Here's the drawing with two shaded views (mm, measured from the low corner). I have some questions. Coordinates: 2 decimals unless noted, no trailing zeros. Write each loop counter-clockwise with the first axis right and the second up, starting at its lowest first coordinate (ties: lowest second). Pieces come first, ordered by that corner, then holes.
Item 1: I want a section at A-A on y = 80.5. Please give me the cut outline in (x, z) (1 decimal).
Item 2: For P1, Ø0.9, axis at y = 75.5, z = 2, coming from the -X side (1 decimal); P2, Ø7, axis at x = 4, y = 23.35, coming from the +Z side; P3, Ø0.9, axis at y = 84, z = 1.5, coming from the +X side, each with a flat end and sliding along its axis, tell me the tip position at first contact or that it passes through.
Item 3: I want a section at B-B on x = 139. Please give me the cut outline in (y, z).
Item 4: If I drill on probe 1 along Y at (x, z) = (155, 1.6) (1 decimal); probe 2 along X at (y, z) = (36.5, 0.25) (1 decimal); probe 3 along X at (y, z) = (42, 1.9) (1 decimal), over which ranges is the centre line in solid material (lowest first)?
Item 5: I want a section at C-C on z = 1.6. State how many separate pieces and enclosed holes the cut face has, then the cut area to 3 significant figures.
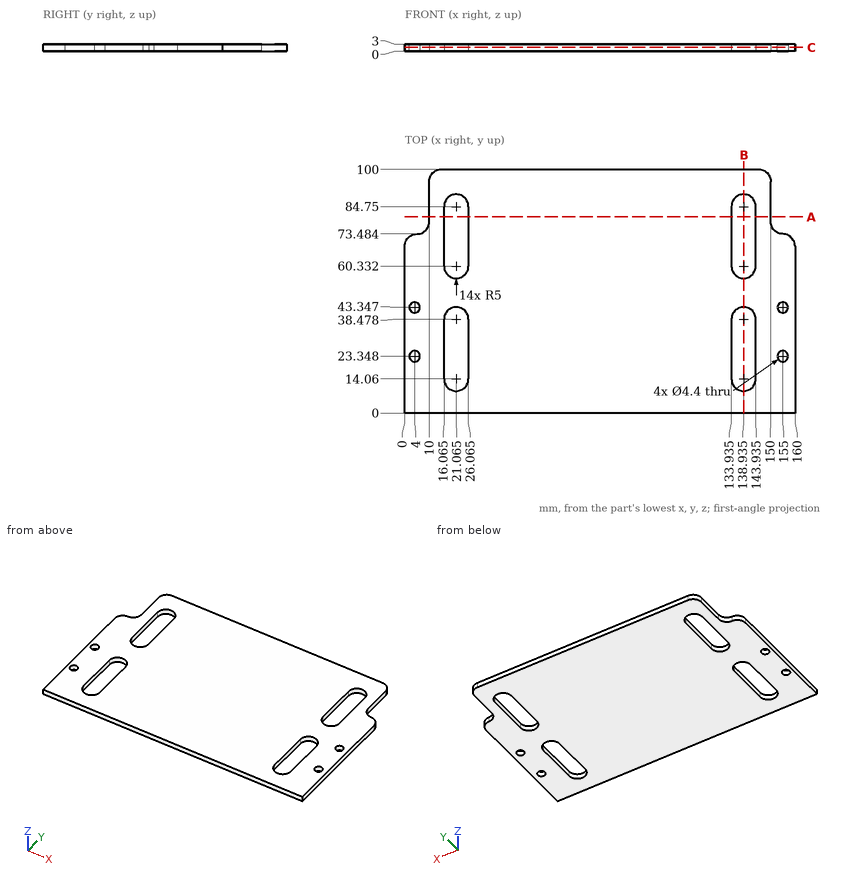
Response values:
1. outline: (10, 0) - (16.1, 0) - (16.1, 3) - (10, 3) - close; (26.1, 0) - (133.9, 0) - (133.9, 3) - (26.1, 3) - close; (143.9, 0) - (150, 0) - (150, 3) - (143.9, 3) - close
2. P1: stops at x = 8.6
2. P2: stops at z = 3
2. P3: stops at x = 150
3. outline: (0, 0) - (9.06, 0) - (9.06, 3) - (0, 3) - close; (43.48, 0) - (55.33, 0) - (55.33, 3) - (43.48, 3) - close; (89.75, 0) - (100, 0) - (100, 3) - (89.75, 3) - close
4. probe 1: y = 0 to 21.1, 25.5 to 41.1, 45.5 to 73.5
4. probe 2: x = 0 to 16.1, 26.1 to 133.9, 143.9 to 160
4. probe 3: x = 0 to 2.3, 5.7 to 17.5, 24.6 to 135.4, 142.5 to 153.3, 156.7 to 160
5. separate pieces: 1
5. enclosed holes: 8
5. area: 14,100 mm2
